Read the model definition and answer for the solid it produces. Units are mm, in the model's axes. A direction names the side the tool comes from. Give positions to 0.01 mm unless a question says otherwise; leave off trailing zeros. Loops run counter-clockwise (first coordinate to the right, second up) from the corner with the lowest first, then second, coordinate; pieces in that order, holes last. Notation, with made-up numbers: (53, -33.5) -> (96, -33.5) arc R28 cw to (96, -15.5) -> close; hole circle Ø1 at (65, 23). An arc over 180 degrees is marked (long way). Return JSON: item names as keys, results as strings. Group by question number.
from build123d import *

# Parameters (mm, degrees)
SALIENTE_EXTRUIR1_DEPTH = 2.6
CROQUIS5_W              = 50
CROQUIS5_H              = 2.6
SALIENTE_EXTRUIR2_DEPTH = 51
REDONDEO1_R             = 5
CROQUIS7_R              = 11
CROQUIS7_R_2            = 1.7
CORTAR_EXTRUIR1_DEPTH   = 77.703340866
CHAFL_N1_SIZE           = 5
CROQUIS8_W              = 2.6
CROQUIS8_H              = 20
SALIENTE_EXTRUIR3_DEPTH = 14.5
CORTAR_EXTRUIR2_DEPTH   = 77.380989945
REDONDEO2_R             = 2.6


with BuildPart() as part:
    # Croquis3 → Saliente-Extruir1 (new body)
    with BuildSketch(Plane.XY):
        Polygon((-25, -27.075), (25, -27.075), (25, 22.075), (20, 27.075), (-20, 27.075), (-25, 22.075), align=None)
        with BuildLine():
            Line((16.9, 15.775), (16.9, -13.775))
            ThreePointArc((16.9, -13.775), (14.7, -15.975), (12.5, -13.775))
            Line((12.5, -13.775), (12.5, 15.775))
            ThreePointArc((12.5, 15.775), (14.7, 17.975), (16.9, 15.775))
        make_face(mode=Mode.SUBTRACT)
        with BuildLine():
            Line((-16.9, 15.775), (-16.9, -13.775))
            ThreePointArc((-16.9, -13.775), (-14.7, -15.975), (-12.5, -13.775))
            Line((-12.5, -13.775), (-12.5, 15.775))
            ThreePointArc((-12.5, 15.775), (-14.7, 17.975), (-16.9, 15.775))
        make_face(mode=Mode.SUBTRACT)
    extrude(amount=SALIENTE_EXTRUIR1_DEPTH)

    # Croquis5 → Saliente-Extruir2 (add)
    with BuildSketch(Plane(origin=(0, 0, 0), x_dir=(-1, 0, 0), z_dir=(0, 0, -1))):
        with Locations((0, -25.775)):
            Rectangle(CROQUIS5_W, CROQUIS5_H)
    extrude(amount=SALIENTE_EXTRUIR2_DEPTH)

    # Redondeo1
    redondeo1_edges = [part.edges().sort_by_distance(p)[0] for p in [
        (0, -27.075, 2.6),
    ]]
    fillet(redondeo1_edges, radius=REDONDEO1_R)

    # Croquis7 → Cortar-Extruir1 (cut, through all)
    with BuildSketch(Plane(origin=(0, -24.475, 0), x_dir=(1, 0, 0), z_dir=(0, 1, 0))):
        with Locations(Location((0, 30, 0), (0, 0, 270))):
            Circle(CROQUIS7_R)
        with Locations(Location((-15.575, 45.875, 0), (0, 0, 270))):
            Circle(CROQUIS7_R_2)
        with Locations(Location((15.575, 45.875, 0), (0, 0, 270))):
            Circle(CROQUIS7_R_2)
        with Locations(Location((15.575, 14.825, 0), (0, 0, 270))):
            Circle(CROQUIS7_R_2)
        with Locations(Location((-15.575, 14.725, 0), (0, 0, 270))):
            Circle(CROQUIS7_R_2)
    extrude(amount=-CORTAR_EXTRUIR1_DEPTH, mode=Mode.SUBTRACT)

    # Chaflán1
    chafl_n1_edges = [part.edges().sort_by_distance(p)[0] for p in [
        (25, -25.775, -51),
        (-25, -25.775, -51),
    ]]
    chamfer(chafl_n1_edges, length=CHAFL_N1_SIZE)

    # Croquis8 → Saliente-Extruir3 (add)
    with BuildSketch(Plane(origin=(0, -24.475, 0), x_dir=(1, 0, 0), z_dir=(0, 1, 0))):
        with Locations((-23.7, 10)):
            Rectangle(CROQUIS8_W, CROQUIS8_H)
        with Locations((23.7, 10)):
            Rectangle(CROQUIS8_W, CROQUIS8_H)
    extrude(amount=SALIENTE_EXTRUIR3_DEPTH)

    # Croquis9 → Cortar-Extruir2 (cut, through all)
    with BuildSketch(Plane.ZY.offset(25)):
        Polygon((-20, -24.475), (-18.827189976, -24.475), (0, -10.965826599), (0, -9.975), (-20, -9.975), align=None)
    extrude(amount=-CORTAR_EXTRUIR2_DEPTH, mode=Mode.SUBTRACT)

    # Redondeo2
    redondeo2_edges = [part.edges().sort_by_distance(p)[0] for p in [
        (0, -24.475, 0),
    ]]
    fillet(redondeo2_edges, radius=REDONDEO2_R)


solid = part.part
1. Section C-C on z = -30 is taken. Determine the outline of the cut face in (x, y) (3 decimals), then the cut area to 3 significant figures.
2. Section D-D on x = 18.5 is taken. Determine the outline of the cut face in (y, z) (3 decimals).
3. Straight lines are drawn through the part: line 1 (X direction, y = -17.5, z = -0.5); line 2 (Y direction, x = -9.5, z = -40.5) (3 decimals); line 3 (Z direction, x = -8.5, y = 3.5). For each, find the intervals that lie inside material, in ascending order. Write a range as from..to.
4. Section A-A on x = 0 is taken. Determine the outline of the cut face in (y, z) (3 decimals).
5. Flat-ended cylindrical pins translate along their axes: pin 1 Ø2 at (x, z) = (-15.575, -45.875) entering from +Y; pin 2 Ø10 at (x, z) = (8, -35.5) entering from +Y (3 decimals); pin 3 Ø2 at (x, y) = (-1.5, -6) entering from -Z. Find the tip coordinate at first contact, or state that the pin passes through.
6. Section B-B on y = 5 is taken. Determine the outline of the cut face in (x, z), then the cut area to 3 significant figures.
7. Which of the six approach directions +Z, -Z, +X, -X, +Y, -Y give full straight-line access (tool end or side, diameter ignored) to faces 4 (the flat face through (12.5, 1, 1)), 5 (the flat face through (11, -24.475, -27)), 6 (the cylindrical face through (-15.064, -25.757, -13.104))?
8. Determine the mould class of faces 1 (the flat face through (23.682, -17.815, -9.545)), 2 (the flat face through (-25, -15, -5)), 3 (the cylindrical face through (14.748, -15.974, 1.282)) for opening direction X: pulls with the +X half, pulls with the -X half, needs draft (parallel to the pull), parting line crosses it, or undercut.
Completed:
{
 "1": {"outline": "(-25, -27.075) -> (-11, -27.075) -> (-11, -24.475) -> (-25, -24.475) -> close; (11, -27.075) -> (25, -27.075) -> (25, -24.475) -> (11, -24.475) -> close", "area": "72.8 mm²"},
 "2": {"outline": "(-27.075, -51) -> (-24.475, -51) -> (-24.475, -2.6) arc R2.6 cw to (-21.875, 0) -> (27.075, 0) -> (27.075, 2.6) -> (-22.075, 2.6) arc R5 ccw to (-27.075, -2.4) -> close"},
 "3": {"line 1": "x = -25..-22.4, 22.4..25", "line 2": "y = -27.075..-24.475", "line 3": "z = 0..2.6"},
 "4": {"outline": "(-27.075, -51) -> (-24.475, -51) -> (-24.475, -41) -> (-27.075, -41) -> close; (-27.075, -19) -> (-24.475, -19) -> (-24.475, -2.6) arc R2.6 cw to (-21.875, 0) -> (27.075, 0) -> (27.075, 2.6) -> (-22.075, 2.6) arc R5 ccw to (-27.075, -2.4) -> close"},
 "5": {"pin 1": "passes through", "pin 2": "stops at y = -24.475", "pin 3": "stops at z = 0"},
 "6": {"outline": "(-25, 0) -> (-16.9, 0) -> (-16.9, 2.6) -> (-25, 2.6) -> close; (-12.5, 0) -> (12.5, 0) -> (12.5, 2.6) -> (-12.5, 2.6) -> close; (16.9, 0) -> (25, 0) -> (25, 2.6) -> (16.9, 2.6) -> close", "area": "107 mm²"},
 "7": {"face 4": "+Z, -Z", "face 5": "-Z, +Y", "face 6": "+Y, -Y"},
 "8": {"face 1": "needs draft", "face 2": "pulls with the -X half", "face 3": "undercut"}
}
